For this review, take the finished solid that the model builds, in its own axes (mm). A direction names the side the tool comes from. Give positions to 0.01 mm unless a question says otherwise; leave off trailing zeros. Write each loop counter-clockwise with the first axis right and the second up, starting at its lowest first coordinate (ties: lowest second). Pieces come first, ordered by that corner, then holes. Notation, with made-up numbers: M 0.25,14 L 21.25,14 A20 ccw 21.25,40 Z; hole C -29.5,79.25 d4. An arc over 180 degrees is marked long. Answer as a JSON object with one key per item and string values. Group by question number.
```python
from build123d import *

# Parameters (mm, degrees)
BOSS_EXTRUDE1_DEPTH = 80
SHELL1_T            = -3
SKETCH3_W           = 46
SKETCH3_H           = 47
BOSS_EXTRUDE2_DEPTH = 17
SKETCH4_W           = 10.2
SKETCH4_H           = 10.2
CUT_EXTRUDE1_DEPTH  = 20
SKETCH6_W           = 15
SKETCH6_H           = 12.8
CUT_EXTRUDE2_DEPTH  = 3
SKETCH7_W           = 40.4
SKETCH7_H           = 50
CUT_EXTRUDE3_DEPTH  = 5
FILLET1_R           = 4
CUT_EXTRUDE7_DEPTH  = 47
SKETCH13_R          = 1.5
CUT_EXTRUDE8_DEPTH  = 25
SKETCH14_R          = 3.1
CUT_EXTRUDE9_DEPTH  = 2
SKETCH17_W          = 45
SKETCH17_H          = 5
BOSS_EXTRUDE5_DEPTH = 74
CUT_EXTRUDE10_REACH = 48.51
SKETCH18_W          = 54
SKETCH18_H          = 45
CUT_EXTRUDE11_REACH = 48.51
SKETCH19_R          = 1.45
BOSS_EXTRUDE6_DEPTH = 47
SKETCH22_R          = 1.45
CUT_EXTRUDE12_DEPTH = 70.509632224
CUT_EXTRUDE13_REACH = 82
SKETCH24_R          = 3.7
SKETCH24_W          = 2
SKETCH24_H          = 3
BOSS_EXTRUDE7_DEPTH = 74
SKETCH27_R          = 1.65
CUT_EXTRUDE14_DEPTH = 10
CUT_EXTRUDE15_START = -3
CUT_EXTRUDE15_DEPTH = 32
CUT_EXTRUDE16_DEPTH = 30
BOSS_EXTRUDE8_DEPTH = 20
SKETCH31_R          = 1.5
CUT_EXTRUDE17_DEPTH = 43.509632224
CUT_EXTRUDE18_DEPTH = 15
CUT_EXTRUDE19_REACH = 48.51
SKETCH33_W          = 10
SKETCH33_H          = 5
SKETCH34_R          = 1.6
CUT_EXTRUDE20_DEPTH = 70.509632224
CUT_EXTRUDE22_DEPTH = 14
CUT_EXTRUDE24_REACH = 5
SKETCH40_R          = 3.7
SKETCH40_W          = 2
SKETCH40_H          = 3


with BuildPart() as part:
    # Sketch2 → Boss-Extrude1 (new body)
    with BuildSketch(Plane(origin=(0, 0, 0), x_dir=(0, 0, -1), z_dir=(1, 0, 0))):
        Polygon((-27.320490368, 20.998248687), (-27.320490368, -29.001751313), (12.679509632, -29.001751313), (12.679509632, -48.511383538), (27.679509632, -48.511383538), (82.679509632, 0.998248687), (82.679509632, 20.998248687), align=None)
    extrude(amount=BOSS_EXTRUDE1_DEPTH)

    # Shell1
    shell1_openings = [part.faces().sort_by_distance(p)[0] for p in [
        (40, 20.998248687, -27.679509632),
    ]]
    offset(amount=SHELL1_T, openings=shell1_openings, kind=Kind.INTERSECTION)

    # Sketch3 → Boss-Extrude2 (add)
    with BuildSketch(Plane(origin=(0, 0, 24.320490368), x_dir=(-1, 0, 0), z_dir=(0, 0, -1))):
        with Locations((-40, -2.501751313)):
            Rectangle(SKETCH3_W, SKETCH3_H)
    extrude(amount=BOSS_EXTRUDE2_DEPTH)

    # Sketch4 → Cut-Extrude1 (cut)
    with BuildSketch(Plane.XY.offset(27.320490368)):
        with Locations((40, -4.001751313)):
            Rectangle(SKETCH4_W, SKETCH4_H)
    extrude(amount=-CUT_EXTRUDE1_DEPTH, mode=Mode.SUBTRACT)

    # Sketch6 → Cut-Extrude2 (cut)
    with BuildSketch(Plane.XZ.offset(29.001751313)):
        with Locations((51.5, 0.920490368)):
            Rectangle(SKETCH6_W, SKETCH6_H)
        with Locations((28.5, 0.920490368)):
            Rectangle(SKETCH6_W, SKETCH6_H)
    extrude(amount=-CUT_EXTRUDE2_DEPTH, mode=Mode.SUBTRACT)

    # Sketch7 → Cut-Extrude3 (cut)
    with BuildSketch(Plane.XY.offset(27.320490368)):
        with Locations((40, -4.001751313)):
            Rectangle(SKETCH7_W, SKETCH7_H)
    extrude(amount=-CUT_EXTRUDE3_DEPTH, mode=Mode.SUBTRACT)

    # Fillet1
    fillet1_edges = [part.edges().sort_by_distance(p)[0] for p in [
        (19.8, -4.001751313, 27.320490368),
        (60.2, -4.001751313, 27.320490368),
        (80, -4.001751313, 27.320490368),
        (0, -4.001751313, 27.320490368),
    ]]
    fillet(fillet1_edges, radius=FILLET1_R)

    # Sketch12 → Cut-Extrude7 (cut)
    with BuildSketch(Plane(origin=(0, 20.998248687, 0), x_dir=(1, 0, 0), z_dir=(0, 1, 0))):
        Polygon((33, -7.320490368), (19.8, -12.320490368), (17, -24.320490368), (17, -7.320490368), align=None)
        Polygon((47, -7.320490368), (63, -7.320490368), (63, -24.320490368), (60.2, -12.320490368), align=None)
    extrude(amount=-CUT_EXTRUDE7_DEPTH, mode=Mode.SUBTRACT)

    # Sketch13 → Cut-Extrude8 (cut)
    with BuildSketch(Plane(origin=(0, 20.998248687, 0), x_dir=(1, 0, 0), z_dir=(0, 1, 0))):
        with Locations((26, -17.320490368)):
            Circle(SKETCH13_R)
        with Locations((54, -17.320490368)):
            Circle(SKETCH13_R)
    extrude(amount=-CUT_EXTRUDE8_DEPTH, mode=Mode.SUBTRACT)

    # Sketch14 → Cut-Extrude9 (cut)
    with BuildSketch(Plane(origin=(0, 20.998248687, 0), x_dir=(1, 0, 0), z_dir=(0, 1, 0))):
        with Locations((26, -17.320490368)):
            Circle(SKETCH14_R)
        with Locations((54, -17.320490368)):
            Circle(SKETCH14_R)
    extrude(amount=-CUT_EXTRUDE9_DEPTH, mode=Mode.SUBTRACT)

    # Sketch17 → Boss-Extrude5 (add)
    with BuildSketch(Plane.ZY.offset(-77)):
        with Locations((-23.179509632, -4.501751313)):
            Rectangle(SKETCH17_W, SKETCH17_H)
    extrude(amount=BOSS_EXTRUDE5_DEPTH)

    # Sketch18 → Cut-Extrude10 (cut, up to next)
    with BuildSketch(Plane(origin=(0, -2.001751313, 0), x_dir=(1, 0, 0), z_dir=(0, 1, 0)), mode=Mode.PRIVATE) as cut_extrude10_sk1:
        with Locations((40, 23.179509632)):
            Rectangle(SKETCH18_W, SKETCH18_H)
    cut_extrude10_tool1 = extrude(cut_extrude10_sk1.sketch, amount=-CUT_EXTRUDE10_REACH, mode=Mode.PRIVATE) & part.part
    add(cut_extrude10_tool1.solids().sort_by_distance((40, -2.001751, -23.17951))[0], mode=Mode.SUBTRACT)

    # Sketch19 → Cut-Extrude11 (cut, up to next)
    with BuildSketch(Plane(origin=(0, -2.001751313, 0), x_dir=(1, 0, 0), z_dir=(0, 1, 0)), mode=Mode.PRIVATE) as cut_extrude11_sk1:
        with Locations((72, 37.179509632)):
            Circle(SKETCH19_R)
    cut_extrude11_tool1 = extrude(cut_extrude11_sk1.sketch, amount=-CUT_EXTRUDE11_REACH, mode=Mode.PRIVATE) & part.part
    add(cut_extrude11_tool1.solids().sort_by_distance((72, -2.001751, -37.17951))[0], mode=Mode.SUBTRACT)
    # Sketch19 → Cut-Extrude11 (cut, up to next)
    with BuildSketch(Plane(origin=(0, -2.001751313, 0), x_dir=(1, 0, 0), z_dir=(0, 1, 0)), mode=Mode.PRIVATE) as cut_extrude11_sk2:
        with Locations((72, 6.179509632)):
            Circle(SKETCH19_R)
    cut_extrude11_tool2 = extrude(cut_extrude11_sk2.sketch, amount=-CUT_EXTRUDE11_REACH, mode=Mode.PRIVATE) & part.part
    add(cut_extrude11_tool2.solids().sort_by_distance((72, -2.001751, -6.17951))[0], mode=Mode.SUBTRACT)
    # Sketch19 → Cut-Extrude11 (cut, up to next)
    with BuildSketch(Plane(origin=(0, -2.001751313, 0), x_dir=(1, 0, 0), z_dir=(0, 1, 0)), mode=Mode.PRIVATE) as cut_extrude11_sk3:
        with Locations((8, 33.179509632)):
            Circle(SKETCH19_R)
    cut_extrude11_tool3 = extrude(cut_extrude11_sk3.sketch, amount=-CUT_EXTRUDE11_REACH, mode=Mode.PRIVATE) & part.part
    add(cut_extrude11_tool3.solids().sort_by_distance((8, -2.001751, -33.17951))[0], mode=Mode.SUBTRACT)
    # Sketch19 → Cut-Extrude11 (cut, up to next)
    with BuildSketch(Plane(origin=(0, -2.001751313, 0), x_dir=(1, 0, 0), z_dir=(0, 1, 0)), mode=Mode.PRIVATE) as cut_extrude11_sk4:
        with Locations((8, 6.179509632)):
            Circle(SKETCH19_R)
    cut_extrude11_tool4 = extrude(cut_extrude11_sk4.sketch, amount=-CUT_EXTRUDE11_REACH, mode=Mode.PRIVATE) & part.part
    add(cut_extrude11_tool4.solids().sort_by_distance((8, -2.001751, -6.17951))[0], mode=Mode.SUBTRACT)

    # Sketch21 → Boss-Extrude6 (add)
    with BuildSketch(Plane(origin=(0, -26.001751313, 0), x_dir=(1, 0, 0), z_dir=(0, 1, 0))):
        Polygon((3, -24.320490368), (3, -14.320490368), (19.333333333, -14.320490368), (17, -24.320490368), align=None)
    extrude(amount=BOSS_EXTRUDE6_DEPTH)

    # Sketch22 → Cut-Extrude12 (cut, through all)
    with BuildSketch(Plane(origin=(0, 20.998248687, 0), x_dir=(1, 0, 0), z_dir=(0, 1, 0))):
        with Locations((10, -19.320490368)):
            Circle(SKETCH22_R)
    extrude(amount=-CUT_EXTRUDE12_DEPTH, mode=Mode.SUBTRACT)

    # Sketch24 → Cut-Extrude13 (cut, up to next)
    with BuildSketch(Plane(origin=(80, 0, 0), x_dir=(0, 0, -1), z_dir=(1, 0, 0)), mode=Mode.PRIVATE) as cut_extrude13_sk1:
        with Locations((26.679509632, -30.511383538)):
            Circle(SKETCH24_R)
    cut_extrude13_tool1 = extrude(cut_extrude13_sk1.sketch, amount=-CUT_EXTRUDE13_REACH, mode=Mode.PRIVATE) & part.part
    add(cut_extrude13_tool1.solids().sort_by_distance((80, -30.511384, -26.67951))[0], mode=Mode.SUBTRACT)
    # Sketch24 → Cut-Extrude13 (cut, up to next)
    with BuildSketch(Plane(origin=(80, 0, 0), x_dir=(0, 0, -1), z_dir=(1, 0, 0)), mode=Mode.PRIVATE) as cut_extrude13_sk2:
        with Locations((34.379509632, -30.511383538)):
            Rectangle(SKETCH24_W, SKETCH24_H)
    cut_extrude13_tool2 = extrude(cut_extrude13_sk2.sketch, amount=-CUT_EXTRUDE13_REACH, mode=Mode.PRIVATE) & part.part
    add(cut_extrude13_tool2.solids().sort_by_distance((80, -30.511384, -34.37951))[0], mode=Mode.SUBTRACT)

    # Sketch26 → Boss-Extrude7 (add)
    with BuildSketch(Plane(origin=(3, 0, 0), x_dir=(0, 0, -1), z_dir=(1, 0, 0))):
        Polygon((79.679509632, 2.334161996), (63.679509632, 2.334161996), (63.679509632, -12.068640106), align=None)
    extrude(amount=BOSS_EXTRUDE7_DEPTH)

    # Sketch27 → Cut-Extrude14 (cut)
    with BuildSketch(Plane(origin=(0, 2.334161996, 0), x_dir=(1, 0, 0), z_dir=(0, 1, 0))):
        with Locations((6, 76.679509632)):
            Circle(SKETCH27_R)
        with Locations((74, 76.679509632)):
            Circle(SKETCH27_R)
    extrude(amount=-CUT_EXTRUDE14_DEPTH, mode=Mode.SUBTRACT)

    # Sketch28 → Cut-Extrude15 (cut)
    with BuildSketch(Plane(origin=(0, 2.334161996, 0), x_dir=(1, 0, 0), z_dir=(0, 1, 0)).offset(CUT_EXTRUDE15_START)):
        Polygon((74, 79.929509632), (71.185417438, 78.304509632), (71.185417438, 75.054509632), (74, 73.429509632), (76.814582562, 75.054509632), (76.814582562, 78.304509632), align=None)
        Polygon((6, 73.429509632), (8.814582562, 75.054509632), (8.814582562, 78.304509632), (6, 79.929509632), (3.185417438, 78.304509632), (3.185417438, 75.054509632), align=None)
    extrude(amount=-CUT_EXTRUDE15_DEPTH, mode=Mode.SUBTRACT)

    # Sketch29 → Cut-Extrude16 (cut)
    with BuildSketch(Plane.XZ.offset(29.001751313)):
        Polygon((7.185417438, 17.695490368), (10, 16.070490368), (12.814582562, 17.695490368), (12.814582562, 20.945490368), (10, 22.570490368), (7.185417438, 20.945490368), align=None)
    extrude(amount=-CUT_EXTRUDE16_DEPTH, mode=Mode.SUBTRACT)

    # Sketch30 → Boss-Extrude8 (add)
    with BuildSketch(Plane(origin=(0, -26.001751313, 0), x_dir=(1, 0, 0), z_dir=(0, 1, 0))):
        Polygon((77, -24.320490368), (63, -24.320490368), (60.2, -12.320490368), (77, -12.320490368), align=None)
    extrude(amount=BOSS_EXTRUDE8_DEPTH)

    # Sketch31 → Cut-Extrude17 (cut, through all)
    with BuildSketch(Plane(origin=(0, -6.001751313, 0), x_dir=(1, 0, 0), z_dir=(0, 1, 0))):
        with Locations((72, -21.320490368)):
            Circle(SKETCH31_R)
    extrude(amount=-CUT_EXTRUDE17_DEPTH, mode=Mode.SUBTRACT)

    # Sketch32 → Cut-Extrude18 (cut)
    with BuildSketch(Plane.XZ.offset(29.001751313)):
        Polygon((72, 24.570490368), (69.185417438, 22.945490368), (69.185417438, 19.695490368), (72, 18.070490368), (74.814582562, 19.695490368), (74.814582562, 22.945490368), align=None)
    extrude(amount=-CUT_EXTRUDE18_DEPTH, mode=Mode.SUBTRACT)

    # Sketch33 → Cut-Extrude19 (cut, up to next)
    with BuildSketch(Plane(origin=(0, -2.001751313, 0), x_dir=(1, 0, 0), z_dir=(0, 1, 0)), mode=Mode.PRIVATE) as cut_extrude19_sk1:
        with Locations((72, 43.179509632)):
            Rectangle(SKETCH33_W, SKETCH33_H)
    cut_extrude19_tool1 = extrude(cut_extrude19_sk1.sketch, amount=-CUT_EXTRUDE19_REACH, mode=Mode.PRIVATE) & part.part
    add(cut_extrude19_tool1.solids().sort_by_distance((72, -2.001751, -43.17951))[0], mode=Mode.SUBTRACT)

    # Sketch34 → Cut-Extrude20 (cut, through all)
    with BuildSketch(Plane(origin=(0, 20.998248687, 0), x_dir=(1, 0, 0), z_dir=(0, 1, 0))):
        with Locations((40, -17.320490368)):
            Circle(SKETCH34_R)
    extrude(amount=-CUT_EXTRUDE20_DEPTH, mode=Mode.SUBTRACT)

    # Sketch36 → Cut-Extrude22 (cut)
    with BuildSketch(Plane.XZ.offset(29.001751313)):
        Polygon((38.375, 20.13507293), (36.75, 17.320490368), (38.375, 14.505907805), (41.625, 14.505907805), (43.25, 17.320490368), (41.625, 20.13507293), align=None)
    extrude(amount=-CUT_EXTRUDE22_DEPTH, mode=Mode.SUBTRACT)

    # Sketch40 → Cut-Extrude24 (cut, up to next)
    with BuildSketch(Plane(origin=(3, 0, 0), x_dir=(0, 0, -1), z_dir=(1, 0, 0)), mode=Mode.PRIVATE) as cut_extrude24_sk1:
        with Locations((26.679509632, -30.511383538)):
            Circle(SKETCH40_R)
    cut_extrude24_tool1 = extrude(cut_extrude24_sk1.sketch, amount=-CUT_EXTRUDE24_REACH, mode=Mode.PRIVATE) & part.part
    add(cut_extrude24_tool1.solids().sort_by_distance((3, -30.511384, -26.67951))[0], mode=Mode.SUBTRACT)
    # Sketch40 → Cut-Extrude24 (cut, up to next)
    with BuildSketch(Plane(origin=(3, 0, 0), x_dir=(0, 0, -1), z_dir=(1, 0, 0)), mode=Mode.PRIVATE) as cut_extrude24_sk2:
        with Locations((18.979509632, -30.511383538)):
            Rectangle(SKETCH40_W, SKETCH40_H)
    cut_extrude24_tool2 = extrude(cut_extrude24_sk2.sketch, amount=-CUT_EXTRUDE24_REACH, mode=Mode.PRIVATE) & part.part
    add(cut_extrude24_tool2.solids().sort_by_distance((3, -30.511384, -18.97951))[0], mode=Mode.SUBTRACT)


solid = part.part
```
Item 1: Insertion check: P1, Ø2.5, axis at x = 54, z = 17.32, coming from the +Y side; P2, Ø8, axis at x = 15.5, z = -67, coming from the +Y side; P3, Ø8.5, axis at x = 65.5, y = -16.5, coming from the -Z side; P4, Ø3.5, axis at y = -3, z = -77, coming from the -X side. Each pin has a flat end and moves straight along its axis. Give the tip position at first contact, or say it passes through.
Item 2: Consider section A-A (x = 40). State how many separate pieces and enclosed holes the cut face has, plus the area to 3 significant figures.
Item 3: Machinability: for faces 1 (the flat face through (28, -28, -5.48)), 2 (the flat face through (37.551, -22.1, 15.933)), 3 (the cylindrical face through (54.692, 7.659, 18.651)), which of the approach directions +Z, -Z, +X, -X, +Y, -Y give a long, thin tool a straight path to every point of the face, cutting with its end or side? Answer none if there is none.
Item 4: Consider section C-C (y = 7). Give the boundary of the cut face in (x, z), plus the area to 3 significant figures.
Item 5: Consider section B-B (x = 49). Give the boundary of the cut face in (y, z).
Item 6: To check wall thickness, follow probe 1 along Z at (x, y) = (26, 1); probe 2 along X at (y, z) = (-3.5, -42.5); probe 3 along X at (y, z) = (15.5, -73). State the ranges of each line that lie inside material, in increasing order.
Item 7: Consider section D-D (z = -55). Give the boundary of the cut face in (x, y).
Item 8: Draft analysis for pull direction Z (two halves, no side actions). For faces 4 (the flat face through (40, 2, 22.32)), 5 (the flat face through (43, 20.998, 9)), 6 (the cylindrical face through (73.64, 0.86, -75.07)), state which applies: released by +Z, released by -Z, zero draft, split by the parting line, or undercut.
Result set:
{
 "1": {"P1": "stops at y = -4", "P2": "stops at y = 2.33", "P3": "stops at z = -67.96", "P4": "stops at x = 0"},
 "2": {"separate pieces": "4", "enclosed holes": "0", "area": "989 mm^2"},
 "3": {"face 1": "+Y, -Y", "face 2": "-Y", "face 3": "+Y"},
 "4": {"outline": "M 0,-82.68 L 80,-82.68 L 80,23.32 A4 ccw 76,27.32 L 64.2,27.32 A4 ccw 60.2,23.32 L 60.2,22.32 L 19.8,22.32 L 19.8,23.32 A4 ccw 15.8,27.32 L 4,27.32 A4 ccw 0,23.32 Z; hole M 3,-79.68 L 77,-79.68 L 77,24.32 L 63,24.32 L 60.2,12.32 L 47,7.32 L 33,7.32 L 19.8,12.32 L 19.33,14.32 L 3,14.32 Z; hole C 10,19.32 d2.9; hole C 26,17.32 d3; hole C 40,17.32 d3.2; hole C 54,17.32 d3", "area": "1,670 mm^2"},
 "5": {"outline": "M -48.51,-27.68 L 1,-82.68 L 21,-82.68 L 21,-79.68 L 2.33,-79.68 L 2.33,-63.68 L -12.07,-63.68 L -45.51,-26.53 L -45.51,-15.68 L -26,-15.68 L -26,-5.48 L -29,-5.48 L -29,-12.68 L -48.51,-12.68 Z; M -29,7.32 L -26,7.32 L -26,8.08 L 21,8.08 L 21,22.32 L -29,22.32 Z"},
 "6": {"probe 1": "z = -82.68 to -63.68, 9.97 to 15.82, 18.82 to 22.32", "probe 2": "x = 0 to 13, 77 to 80", "probe 3": "x = 0 to 3, 77 to 80"},
 "7": {"outline": "M 0,-23.92 L 80,-23.92 L 80,21 L 77,21 L 77,-19.88 L 3,-19.88 L 3,21 L 0,21 Z"},
 "8": {"face 4": "released by +Z", "face 5": "zero draft", "face 6": "undercut"}
}
